Could you check a few things on this model? Use its own coordinates, in mm. A direction names the side the tool comes from. Give positions to 0.01 mm unless a question says otherwise; leave off trailing zeros. Loops run counter-clockwise (first coordinate to the right, second up) from the corner with the lowest first, then second, coordinate; pieces in that order, holes last. Notation, with made-up numbers: (63.5, 46.5) -> (89.5, 46.5) arc R29 cw to (89.5, 74.5) -> close; hole circle Ø4 at (3.5, 85.25). An arc over 180 degrees is marked (long way). Write each question's results on one line, items separated by ' | '. Start each with the question number.
Q1. Which directions (+Z, -Z, +X, -X, +Y, -Y) give clear straight access to the entire face, cutting with the end or side of a thin tool? Please do faces 1 (the face through (10, 8, 3)), 2 (the face through (-1.85, 23.75, -5.89)), 3 (the face through (-7.167, 22.74, -4.57)).
Q2. Will these pins go through, and if not, where does the flat tip stop? P1, Ø12, axis at x = 5.5, y = 16, coming from the +Z side; P2, Ø1, axis at y = 18.5, z = 3, coming from the +X side; P3, Ø1.5, axis at y = 12.5, z = 7, coming from the +X side.
Q3. If we section it at A-A, the plane y = 2.75: List the corners of the cut face in (x, z) for me, plus the area to 3 significant figures.
Q4. If I drill on line 1 along X through (y, z) = (1.75, 1.5); line 2 along Z through (x, y) = (0, 23.8) (3 decimals); line 3 along X through (y, z) = (7.25, 3.75), over which ranges is the centre line in solid material (lowest first)?
Q5. If we section it at B-B, the plane y = 20.5: List the corners of the cut face in (x, z) for me, plus the area to 3 significant figures.
Q6. We'd pull the mould along Y, two halves only. Please class faces 4 (the face through (4, 4, 9)), 5 (the face through (4, 5.7, -9)), 6 (the face through (8.437, 17.249, -4.388)), 7 (the face through (10.787, 8.986, 2.395)): released by +Y, released by -Y, zero draft, split by the parting line, or undercut.
from build123d import *

# Parameters (mm, degrees)
CHAMFER_1_SIZE = 1
CHAMFER_2_SIZE = 0.5
FILLET_1_R     = 0.3
CHAMFER_3_SIZE = 0.5


with BuildPart() as part:
    # 스케치1 → 회전1 (revolve)
    with BuildSketch(Plane(origin=(0, 0, 0), x_dir=(0, 0, -1), z_dir=(1, 0, 0))):
        with BuildLine():
            Line((7.1, 0), (7.1, 23))
            Line((7.1, 23), (6.175, 23))
            Line((6.175, 23), (6.175, 24))
            Line((6.175, 24), (8.5, 24))
            Line((8.5, 24), (8.5, 22))
            Line((8.5, 22), (11.05, 10))
            Line((11.05, 10), (11.05, 8))
            Line((11.05, 8), (10.05, 8))
            Line((10.05, 8), (10.05, 5.7))
            Line((10.05, 5.7), (9.55, 5.7))
            ThreePointArc((9.55, 5.7), (8.7, 4.85), (9.55, 4))
            Line((9.55, 4), (10.05, 4))
            Line((10.05, 4), (10.05, 0))
            Line((10.05, 0), (7.1, 0))
        make_face()
    revolve(axis=Axis((0, 0, 0), (0, 1, 0)))

    # 모따기1
    chamfer_1_edges = [part.edges().sort_by_distance(p)[0] for p in [
        (0, 0, 10.05),
    ]]
    chamfer(chamfer_1_edges, length=CHAMFER_1_SIZE)

    # 모따기2
    chamfer_2_edges = [part.edges().sort_by_distance(p)[0] for p in [
        (0, 24, 8.5),
    ]]
    chamfer(chamfer_2_edges, length=CHAMFER_2_SIZE)

    # 필렛1
    fillet_1_edges = [part.edges().sort_by_distance(p)[0] for p in [
        (0, 0, 7.1),
    ]]
    fillet(fillet_1_edges, radius=FILLET_1_R)

    # 모따기3
    chamfer_3_edges = [part.edges().sort_by_distance(p)[0] for p in [
        (0, 23, 6.175),
    ]]
    chamfer(chamfer_3_edges, length=CHAMFER_3_SIZE)


solid = part.part
Final values:
1) face 1: -Y | face 2: +Y, -Y | face 3: +Y
2) P1: stops at z = 10.63 | P2: stops at x = 8.94 | P3: stops at x = 8.49
3) outline: circle Ø20.1 at (0, 0); hole circle Ø14.2 at (0, 0) | area: 159 mm²
4) line 1: x = -9.94 to -6.94, 6.94 to 9.94 | line 2: z = -8.2 to -6.175, 6.175 to 8.2 | line 3: x = -9.32 to -6.03, 6.03 to 9.32
5) outline: circle Ø17.64 at (0, 0); hole circle Ø14.2 at (0, 0) | area: 86.0 mm²
6) face 4: undercut | face 5: undercut | face 6: released by +Y | face 7: zero draft
